from build123d import *
from OCP.BRepFilletAPI import BRepFilletAPI_MakeChamfer

# Parameters (mm, degrees)
SKICA1_R                = 12.5
SKICA1_R_2              = 1.5
P_IDAT_VYSUNUT_M1_DEPTH = 2
ZKOSEN_1_SIZE           = 0.8
ZKOSEN_1_SIZE2          = 1.385640646


with BuildPart() as part:
    # Skica1 → Přidat vysunutím1 (new body)
    with BuildSketch(Plane.XY):
        with BuildLine():
            Line((6.363961031, 30.405591591), (30.405591591, 6.363961031))
            ThreePointArc((30.405591591, 6.363961031), (31.577164466, 3.535533906), (30.405591591, 0.707106781))
            Line((30.405591591, 0.707106781), (8.485281374, -21.213203436))
            ThreePointArc((8.485281374, -21.213203436), (4.498831017, -23.654503108), (-0.161661635, -24.01718587))
            Line((-0.161661635, -24.01718587), (-18.229225849, -21.133937116))
            ThreePointArc((-18.229225849, -21.133937116), (-20.152543264, -20.152543264), (-21.133937116, -18.229225849))
            Line((-21.133937116, -18.229225849), (-24.01718587, -0.161661635))
            ThreePointArc((-24.01718587, -0.161661635), (-23.654503108, 4.498831017), (-21.213203436, 8.485281374))
            Line((-21.213203436, 8.485281374), (0.707106781, 30.405591591))
            ThreePointArc((0.707106781, 30.405591591), (3.535533906, 31.577164466), (6.363961031, 30.405591591))
        make_face()
        Circle(SKICA1_R, mode=Mode.SUBTRACT)
        with Locations((0, 16)):
            Circle(SKICA1_R_2, mode=Mode.SUBTRACT)
        with Locations((16, 0)):
            Circle(SKICA1_R_2, mode=Mode.SUBTRACT)
        with Locations((0, -16)):
            Circle(SKICA1_R_2, mode=Mode.SUBTRACT)
        with Locations((-16, 0)):
            Circle(SKICA1_R_2, mode=Mode.SUBTRACT)
        with Locations((-17.67766953, -17.67766953)):
            Circle(SKICA1_R_2, mode=Mode.SUBTRACT)
        with Locations((27.577164466, 3.535533906)):
            Circle(SKICA1_R_2, mode=Mode.SUBTRACT)
        with Locations(Location((3.535533906, 27.577164466, 0), (0, 0, 180))):
            Circle(SKICA1_R_2, mode=Mode.SUBTRACT)
    extrude(amount=P_IDAT_VYSUNUT_M1_DEPTH)

    # Zkosení1: one chamfer whose edges measure the first distance from different faces: ONE call of the kernel's chamfer builder (chamfer() names one face for all edges)
    zkosen_1_edges_1 = [part.edges().sort_by_distance(p)[0] for p in [
        (-1.5, 16, 0),
    ]]
    zkosen_1_side_1 = [part.faces().sort_by_distance(p)[0] for p in [
        (-1.5, 16, 1),
    ]]
    zkosen_1_edges_2 = [part.edges().sort_by_distance(p)[0] for p in [
        (14.5, 0, 0),
    ]]
    zkosen_1_side_2 = [part.faces().sort_by_distance(p)[0] for p in [
        (14.5, 0, 1),
    ]]
    zkosen_1_edges_3 = [part.edges().sort_by_distance(p)[0] for p in [
        (-1.5, -16, 0),
    ]]
    zkosen_1_side_3 = [part.faces().sort_by_distance(p)[0] for p in [
        (-1.5, -16, 1),
    ]]
    zkosen_1_edges_4 = [part.edges().sort_by_distance(p)[0] for p in [
        (-17.5, 0, 0),
    ]]
    zkosen_1_side_4 = [part.faces().sort_by_distance(p)[0] for p in [
        (-17.5, 0, 1),
    ]]
    zkosen_1 = BRepFilletAPI_MakeChamfer(part.part.solid().wrapped)
    for e in zkosen_1_edges_1:
        zkosen_1.Add(ZKOSEN_1_SIZE, ZKOSEN_1_SIZE2, e.wrapped, zkosen_1_side_1[0].wrapped)  # the first distance lies on this face
    for e in zkosen_1_edges_2:
        zkosen_1.Add(ZKOSEN_1_SIZE, ZKOSEN_1_SIZE2, e.wrapped, zkosen_1_side_2[0].wrapped)  # the first distance lies on this face
    for e in zkosen_1_edges_3:
        zkosen_1.Add(ZKOSEN_1_SIZE, ZKOSEN_1_SIZE2, e.wrapped, zkosen_1_side_3[0].wrapped)  # the first distance lies on this face
    for e in zkosen_1_edges_4:
        zkosen_1.Add(ZKOSEN_1_SIZE, ZKOSEN_1_SIZE2, e.wrapped, zkosen_1_side_4[0].wrapped)  # the first distance lies on this face
    add(Compound.cast(zkosen_1.Shape()), mode=Mode.REPLACE)


solid = part.part
Can you work these out from the model? Positions are in its coordinate system, mm. Give positions to 0.01 mm unless a question says otherwise; leave off trailing zeros. Loops run counter-clockwise (first coordinate to the right, second up) from the corner with the lowest first, then second, coordinate; pieces in that order, holes last. Notation, with made-up numbers: (25.25, 74) -> (60.25, 74) arc R28 ccw to (60.25, 101) -> close; hole circle Ø10 at (7.25, 44.25). An arc over 180 degrees is marked (long way). Write item = value, one per line.
1) Suppose I cut it at D-D on x = -5. Write out the boundary of the cut face in (y, z), then the cut area to 3 significant figures.
Check result:
outline = (-23.25, 0) -> (-11.46, 0) -> (-11.46, 2) -> (-23.25, 2) -> close; (11.46, 0) -> (24.7, 0) -> (24.7, 2) -> (11.46, 2) -> close
area = 50.1 mm2
2) Suppose I cut it at A-A on x = 4. Write out the boundary of the cut face in (y, z).
Check result:
outline = (-23.8, 0) -> (-11.84, 0) -> (-11.84, 2) -> (-23.8, 2) -> close; (11.84, 0) -> (26.15, 0) -> (26.15, 2) -> (11.84, 2) -> close; (29, 0) -> (31.55, 0) -> (31.55, 2) -> (29, 2) -> close
3) I need wall thicknesses on L1, parallel to X at y = -17, z = 1.15; L2, parallel to Y at x = 0, z = 1.4; L3, parallel to Y at x = -4, z = 0.95. Which ranges of each line are inside material? Lowest first, please. Write a range as from..to.
Check result:
L1 = -21.33..-19.02, -16.34..-1.12, 1.12..12.7
L2 = -24.04..-17.5, -14.5..-12.5, 12.5..14.5, 17.5..29.7
L3 = -23.4..-11.84, 11.84..25.7
4) Suppose I cut it at B-B on y = 16. Write out the boundary of the cut face in (x, z), then the cut area to 3 significant figures.
Check result:
outline = (-13.7, 0) -> (-2.89, 0) -> (-1.5, 0.8) -> (-1.5, 2) -> (-13.7, 2) -> close; (1.5, 0.8) -> (2.89, 0) -> (20.77, 0) -> (20.77, 2) -> (1.5, 2) -> close
area = 61.8 mm2
5) Suppose I cut it at C-C on z = 1.5. Give the number of separate pieces and of enclosed holes in the cut face, then the cut area to 3 significant figures.
Check result:
separate_pieces = 1
enclosed_holes = 8
area = 1,450 mm2
6) Thinking about a two-plate mould opening in X: for faces 1 (the cylindrical face through (27.382, 5.023, 0.986)), 2 (the cylindrical face through (3.86, 29.04, 0.99)), 3 (the cylindrical face through (31.577, 3.58, 0.986)), 4 (the flat face through (-9.069, -22.596, 0.986)), which applies, released by +X, released by -X, zero draft, split by the parting line, or undercut?
Check result:
face_1 = undercut
face_2 = undercut
face_3 = released by +X
face_4 = released by -X
